Could you check a few things on this drawing? It's one solid part, dimensions in mm from its lowest x, y, z. Give positions to 0.01 mm unless a question says otherwise; leave off trailing zeros. Order: outer loops, then holes, each group sorted by start corner. A loop starts at its lowest first (then second) coordinate and runs counter-clockwise, first axis right, second up.
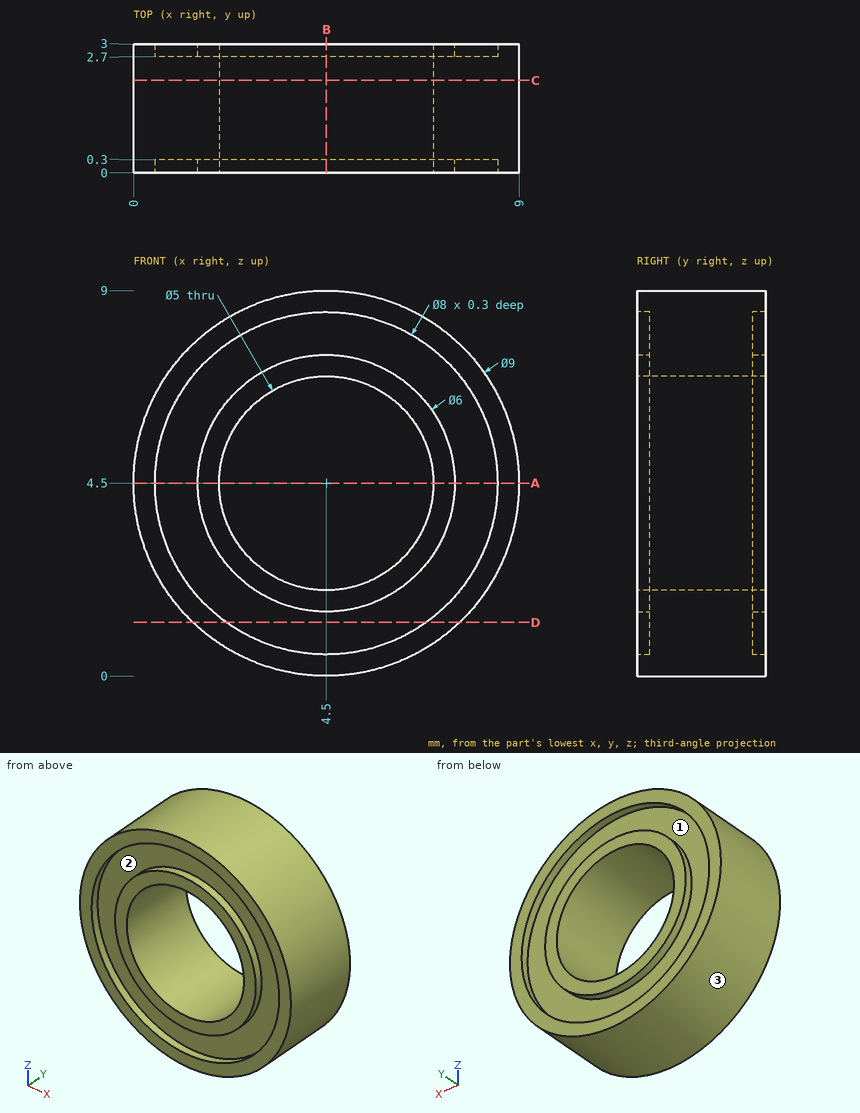
Item 1: Please list where these lines run through material, in increasing order: line 1 along X through (y, z) = (0.2, 4.5); line 2 along X through (y, z) = (1.6, 4.5).
Findings:
line 1: x = 0 to 0.5, 1.5 to 2, 7 to 7.5, 8.5 to 9
line 2: x = 0 to 2, 7 to 9
Item 2: Imagine slicing it at B-B on x = 4.5. List the corners of the cut face in (y, z) for me.
Findings:
outline: (0, 0) - (3, 0) - (3, 0.5) - (2.7, 0.5) - (2.7, 1.5) - (3, 1.5) - (3, 2) - (0, 2) - (0, 1.5) - (0.3, 1.5) - (0.3, 0.5) - (0, 0.5) - close; (0, 7) - (3, 7) - (3, 7.5) - (2.7, 7.5) - (2.7, 8.5) - (3, 8.5) - (3, 9) - (0, 9) - (0, 8.5) - (0.3, 8.5) - (0.3, 7.5) - (0, 7.5) - close
Item 3: Imagine slicing it at D-D on z = 1.25. List the corners of the cut face in (x, y) for me.
Findings:
outline: (1.39, 0) - (2.17, 0) - (2.17, 0.3) - (6.83, 0.3) - (6.83, 0) - (7.61, 0) - (7.61, 3) - (6.83, 3) - (6.83, 2.7) - (2.17, 2.7) - (2.17, 3) - (1.39, 3) - close
Item 4: Imagine slicing it at C-C on y = 2.15. List the corners of the cut face in (x, z) for me.
Findings:
outline: circle Ø9 at (4.5, 4.5); hole circle Ø5 at (4.5, 4.5)
Item 5: We'd pull the mould along X, two halves only. Please class the marked faces 1, 2 and 3: +X half, -X half, draft (parallel to the pull), parting line (faces both ways), or undercut.
Findings:
face 1: undercut
face 2: undercut
face 3: parting line
Item 6: Imagine slicing it at A-A on z = 4.5. List the corners of the cut face in (x, y) for me, then the cut area to 3 significant figures.
Findings:
outline: (0, 0) - (0.5, 0) - (0.5, 0.3) - (1.5, 0.3) - (1.5, 0) - (2, 0) - (2, 3) - (1.5, 3) - (1.5, 2.7) - (0.5, 2.7) - (0.5, 3) - (0, 3) - close; (7, 0) - (7.5, 0) - (7.5, 0.3) - (8.5, 0.3) - (8.5, 0) - (9, 0) - (9, 3) - (8.5, 3) - (8.5, 2.7) - (7.5, 2.7) - (7.5, 3) - (7, 3) - close
area: 10.8 mm2
Item 7: For pin 1 (1.5 mm diameter, centred on y = 0.5, z = 3, fed in from -X); pin 2 (1.5 mm diameter, centred on y = 1, z = 1, fed in from -X), each with a flat end and sliding along its axis, tell me the tip position at first contact or that it passes through.
Findings:
pin 1: stops at x = 0.06
pin 2: stops at x = 0.94
